```python
from build123d import *

# Parameters (mm, degrees)
F0_W     = 609.6
F0_H     = 285.75
F1_DEPTH = 19.05
F2_W     = 12.7
F2_H     = 25.4
F3_DEPTH = 609.601
F4_R     = 31.75
F5_DEPTH = 19.051


with BuildPart() as f1:
    # F0 (on Front) → F1 (new body)
    with BuildSketch(Plane.XZ):
        Rectangle(F0_W, F0_H)
    extrude(amount=F1_DEPTH)

    # F2 (on face) → F3 (cut, through all)
    with BuildSketch(Plane(origin=(-304.8, 0, 0), x_dir=(0, -1, 0), z_dir=(-1, 0, 0))):
        with Locations((6.35, -130.175)):
            Rectangle(F2_W, F2_H)
    extrude(amount=-F3_DEPTH, mode=Mode.SUBTRACT)

    # F4 (on face) → F5 (cut, through all)
    with BuildSketch(Plane.XZ.offset(19.05)):
        with Locations((-190.5, 28.575)):
            Circle(F4_R)
        with Locations((190.5, 28.575)):
            Circle(F4_R)
    extrude(amount=-F5_DEPTH, mode=Mode.SUBTRACT)


solid = f1.part
```
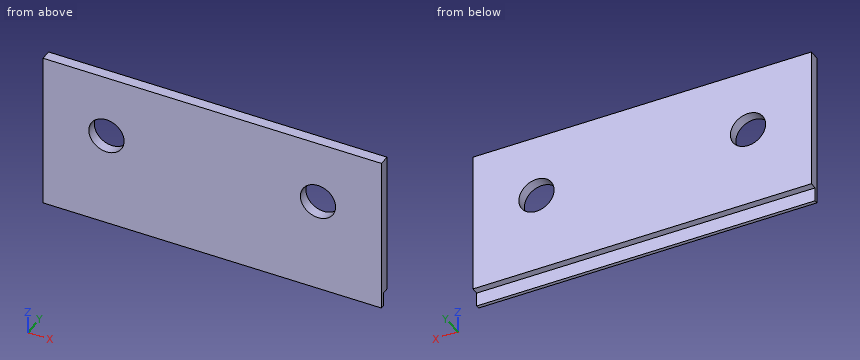
Check sheet for the modelled part. Datum: model origin and axes. Units: mm. Give positions to 0.01 mm unless a question says otherwise; leave off trailing zeros. Order: outer loops, then holes, each group sorted by start corner. A loop starts at its lowest first (then second) coordinate and runs counter-clockwise, first axis right, second up. Notation, with made-up numbers: (-38.5, -5.5) -> (-11.5, -5.5) arc R35 ccw to (-11.5, 27.5) -> close; hole circle Ø8 at (-4, 73). An arc over 180 degrees is marked (long way). Use CSV: the item, a comma, the result in double quotes. Start each with the question number.
1) Material ranges on line 1 (X direction, y = -7, z = 31); line 2 (Z direction, x = -190.5, y = -13.5) (3 decimals); line 3 (Z direction, x = 190.5, y = -10.75) (3 decimals), recorded low to high. Write a range as from..to.
2) Sectioned sample at D-D, the plane x = -267. Record the boundary of the cut face in (y, z) (3 decimals), plus the area to 3 significant figures.
3) Sectioned sample at A-A, the plane x = -190.5. Record the boundary of the cut face in (y, z) (3 decimals).
4) Sectioned sample at C-C, the plane y = -6. Record the boundary of the cut face in (x, z) (3 decimals), plus the area to 3 significant figures.
5) Sectioned sample at B-B, the plane z = 15. Record the boundary of the cut face in (x, y), plus the area to 3 significant figures.
6) Go/stop test with flat-tipped pins: P1, Ø4, axis at x = -222.5, y = -3.5, coming from the -Z side (3 decimals); P2, Ø7.5, axis at x = 122.5, z = -127.5, coming from the +Y side. Record where each tip stops, or that it passes through.
Recorded:
1,line 1,"-304.8..-222.16, -158.84..158.84, 222.16..304.8"
1,line 2,"-142.875..-3.175, 60.325..142.875"
1,line 3,"-117.475..-3.175, 60.325..142.875"
2,outline,"(-19.05, -142.875) -> (-12.7, -142.875) -> (-12.7, -117.475) -> (0, -117.475) -> (0, 142.875) -> (-19.05, 142.875) -> close"
2,area,"5,120 mm2"
3,outline,"(-19.05, -142.875) -> (-12.7, -142.875) -> (-12.7, -117.475) -> (0, -117.475) -> (0, -3.175) -> (-19.05, -3.175) -> close; (-19.05, 60.325) -> (0, 60.325) -> (0, 142.875) -> (-19.05, 142.875) -> close"
4,outline,"(-304.8, -117.475) -> (304.8, -117.475) -> (304.8, 142.875) -> (-304.8, 142.875) -> close; hole circle Ø63.5 at (-190.5, 28.575); hole circle Ø63.5 at (190.5, 28.575)"
4,area,"152,000 mm2"
5,outline,"(-304.8, -19.05) -> (-219.2, -19.05) -> (-219.2, 0) -> (-304.8, 0) -> close; (-161.8, -19.05) -> (161.8, -19.05) -> (161.8, 0) -> (-161.8, 0) -> close; (219.2, -19.05) -> (304.8, -19.05) -> (304.8, 0) -> (219.2, 0) -> close"
5,area,"9,430 mm2"
6,P1,"z = -117.475"
6,P2,"y = -12.7"
